```python
from build123d import *

# Parameters (mm, degrees)
SKETCH1_R           = 1.5
BOSS_EXTRUDE1_DEPTH = 1.6
SKETCH2_W           = 10
SKETCH2_H           = 6
BOSS_EXTRUDE3_DEPTH = 6
SKETCH2_7_W         = 37
SKETCH2_7_H         = 2.5
SKETCH2_7_W_2       = 2.5
SKETCH2_7_H_2       = 26
SKETCH2_7_W_3       = 42
SKETCH2_7_W_4       = 24
BOSS_EXTRUDE4_DEPTH = 8.65


with BuildPart() as part:
    # Sketch1 → Boss-Extrude1 (new body)
    with BuildSketch(Plane(origin=(0, 0, 0), x_dir=(1, 0, 0), z_dir=(0, 1, 0))):
        with BuildLine():
            Line((-32, 33), (32, 33))
            ThreePointArc((32, 33), (34.121320344, 32.121320344), (35, 30))
            Line((35, 30), (35, -30))
            ThreePointArc((35, -30), (34.121320344, -32.121320344), (32, -33))
            Line((32, -33), (-32, -33))
            ThreePointArc((-32, -33), (-34.121320344, -32.121320344), (-35, -30))
            Line((-35, -30), (-35, 30))
            ThreePointArc((-35, 30), (-34.121320344, 32.121320344), (-32, 33))
        make_face()
        with Locations((-32, 30)):
            Circle(SKETCH1_R, mode=Mode.SUBTRACT)
        with Locations((32, 30)):
            Circle(SKETCH1_R, mode=Mode.SUBTRACT)
        with Locations((32, -30)):
            Circle(SKETCH1_R, mode=Mode.SUBTRACT)
        with Locations((-32, -30)):
            Circle(SKETCH1_R, mode=Mode.SUBTRACT)
    extrude(amount=BOSS_EXTRUDE1_DEPTH)

    # Sketch2 → Boss-Extrude3 (add)
    with BuildSketch(Plane(origin=(0, 1.6, 0), x_dir=(1, 0, 0), z_dir=(0, 1, 0))):
        with Locations((11, 26.5)):
            Rectangle(SKETCH2_W, SKETCH2_H)
        with Locations((22, -18.5)):
            Rectangle(SKETCH2_W, SKETCH2_H)
    extrude(amount=BOSS_EXTRUDE3_DEPTH)

    # Sketch2_7 → Boss-Extrude4 (add)
    with BuildSketch(Plane(origin=(0, 1.6, 0), x_dir=(1, 0, 0), z_dir=(0, 1, 0))):
        with Locations((-8, 14)):
            Rectangle(SKETCH2_7_W, SKETCH2_7_H)
        with Locations((19, 7.5)):
            Rectangle(SKETCH2_7_W_2, SKETCH2_7_H_2)
        with Locations((-10.5, -6.25)):
            Rectangle(SKETCH2_7_W_3, SKETCH2_7_H)
        with Locations((1, -13.5)):
            Rectangle(SKETCH2_7_W_4, SKETCH2_7_H)
    extrude(amount=BOSS_EXTRUDE4_DEPTH)


solid = part.part
```
Here's how the part is built. I have some questions about the finished solid (model axes, mm). A direction names the side the tool comes from. Give positions to 0.01 mm unless a question says otherwise; leave off trailing zeros. Write each loop counter-clockwise with the first axis right and the second up, starting at its lowest first coordinate (ties: lowest second). Pieces come first, ordered by that corner, then holes. Notation, with made-up numbers: M 60.5,-7.5 L 99.5,-7.5 A31 ccw 99.5,25.5 Z; hole C 86,16.25 d11. An arc over 180 degrees is marked long. Put each result on its own line as item: value. Start each with the question number.
Item 1: If we section it at B-B, the plane x = -15: Write out the boundary of the cut face in (y, z), then the cut area to 3 significant figures.
Item 2: I need wall thicknesses on L1, parallel to Z at x = -32, y = 0.9; L2, parallel to X at y = 1.15, z = -30; L3, parallel to Z at x = 4, y = 3.5. Which ranges of each line are inside material? Lowest first, please. Write a range as from..to.
Item 3: If we section it at A-A, the plane y = 8.5: Write out the boundary of the cut face in (x, z), then the cut area to 4 significant figures.
Item 4: If we section it at C-C, the plane x = -3.5: Write out the boundary of the cut face in (y, z).
Item 5: Thinking about a two-plate mould opening in Z: for faces 6 (the flat face through (22, 5, 21.5)), 7 (the cylindrical face through (30.89, 0.79, 28.99)), 8 (the flat face through (-11, 6, 14)), which applies, +Z half, -Z half, draft (parallel to the pull), parting line (faces both ways), or undercut?
Item 6: Will these pins go through, and if not, where does the flat tip stop? pin 1 (3 mm diameter, centred on x = 8.5, z = -5.5, fed in from +Y); pin 2 (3 mm diameter, centred on x = 11, y = 3.5, fed in from -Z); pin 3 (1.2 mm diameter, centred on y = 4, z = 6.5, fed in from -X); pin 4 (5 mm diameter, centred on x = 32, z = -30, fed in from -Y).
Item 7: On a 3-axis mill with a long thin cutter (end or side, diameter ignored), from which of +Z, -Z, +X, -X, +Y, -Y can I reach the whole of each face in a straight line? I mean faces 1 (the flat face through (27, 5, 19)), 2 (the flat face through (19, 6, 5.5)), 3 (the flat face through (-11, 6, 5)), 4 (the flat face through (10.5, 6, -14)), 5 (the flat face through (11, 7.6, -27)). Say none if no direction works.
Values:
1. outline: M 0,-33 L 1.6,-33 L 1.6,-15.25 L 10.25,-15.25 L 10.25,-12.75 L 1.6,-12.75 L 1.6,5 L 10.25,5 L 10.25,7.5 L 1.6,7.5 L 1.6,33 L 0,33 Z
1. area: 149 mm²
2. L1: -33..-31.5, -28.5..28.5, 31.5..33
2. L2: -35..-33.5, -30.5..30.5, 33.5..35
2. L3: -15.25..-12.75, 5..7.5, 12.25..14.75
3. outline: M -31.5,5 L 10.5,5 L 10.5,7.5 L -31.5,7.5 Z; M -26.5,-15.25 L 10.5,-15.25 L 10.5,-12.75 L -26.5,-12.75 Z; M -11,12.25 L 13,12.25 L 13,14.75 L -11,14.75 Z; M 17.75,-20.5 L 20.25,-20.5 L 20.25,5.5 L 17.75,5.5 Z
3. area: 322.5 mm²
4. outline: M 0,-33 L 1.6,-33 L 1.6,-15.25 L 10.25,-15.25 L 10.25,-12.75 L 1.6,-12.75 L 1.6,5 L 10.25,5 L 10.25,7.5 L 1.6,7.5 L 1.6,12.25 L 10.25,12.25 L 10.25,14.75 L 1.6,14.75 L 1.6,33 L 0,33 Z
5. face 6: +Z half
5. face 7: undercut
5. face 8: draft
6. pin 1: y = 1.6
6. pin 2: z = -29.5
6. pin 3: x = -31.5
6. pin 4: y = 0
7. face 1: +Z, -Z, +X, +Y
7. face 2: +X, +Y
7. face 3: -X, +Y
7. face 4: +Y
7. face 5: -Z, +X, -X, +Y
